Geometry check sheet. Reference: the model listing, model coordinates, mm. A direction names the side the tool comes from. Coordinates: 2 decimals unless noted, no trailing zeros. Write each loop counter-clockwise with the first axis right and the second up, starting at its lowest first coordinate (ties: lowest second). Pieces come first, ordered by that corner, then holes. Notation, with made-up numbers: (39.5, 14.25) -> (76.5, 14.25) arc R7 ccw to (76.5, 23.25) -> close; hole circle Ø4 at (80.25, -14). An arc over 180 degrees is marked (long way). Answer in a Markdown table with one row per item. Add a question column.
Q1. Gauge pin test, flat ends, axial feed: P1, Ø1.8, axis at x = 10, z = -3.5, coming from the -Y side; P2, Ø5, axis at x = 7.5, y = 9, coming from the -Z side; P3, Ø5, axis at x = 4, z = 3, coming from the -Y side. Record the tip position at first contact, or that the pin passes through.
Q2. Section check B-B, the plane z = -11. Record the boundary of the cut face in (x, y), and give its area (3 significant figures).
Q3. Tool access check on faces 1 (the face through (11, -4.65, -1)), 2 (the face through (6, -1.5, -25)), 3 (the face through (9.65, -6.79, -10.76)), 4 (the face through (6, 0, 2)), 5 (the face through (6, -1.5, 2)). Record the directions out of +Z, -Z, +X, -X, +Y, -Y that give a thin tool (end or side, any length) a straight path to the whole face; none if there is none.
Q4. Section check A-A, the plane x = 10.75. Record the boundary of the cut face in (y, z), and give its area (3 significant figures).
Q5. Section check C-C, the plane y = 13. Record the boundary of the cut face in (x, z), and give its area (3 significant figures).
Q6. Thickness scan on line 1 (Y direction, x = 7.75, z = -1.5); line 2 (Y direction, x = 9.5, z = -14); line 3 (Z direction, x = 3.75, y = -4.5). Record the ranges inside material, lowest first.
```python
from build123d import *

# Parameters (mm, degrees)
EXTRUDE_1_DEPTH = 12
SKETCH_2_R      = 6
EXTRUDE_2_DEPTH = 4.35
SKETCH_3_R      = 1.75
EXTRUDE_3_DEPTH = 4


with BuildPart() as part:
    # 草图1 → 凸台-拉伸1 (new body)
    with BuildSketch(Plane(origin=(0, 0, 0), x_dir=(0, 0, -1), z_dir=(1, 0, 0))):
        Polygon((0, 0), (0, 15), (23, 15), (23, 0), (27.4, 0), (27.4, -1.5), (23, -1.5), (23, -4.65), (0, -4.65), (0, -1.5), (-4.4, -1.5), (-4.4, 0), align=None)
    extrude(amount=EXTRUDE_1_DEPTH)

    # 草图2 → 凸台-拉伸2 (add)
    with BuildSketch(Plane(origin=(0, -4.65, 0), x_dir=(-1, 0, 0), z_dir=(0, -1, 0))):
        with Locations(Location((-6, 6, 0), (0, 0, 270))):
            Circle(SKETCH_2_R)
    extrude(amount=EXTRUDE_2_DEPTH)

    # 草图3 → 凸台-拉伸3 (add)
    with BuildSketch(Plane.XZ.offset(9)):
        with Locations(Location((6, -6, 0), (0, 0, 270))):
            Circle(SKETCH_3_R)
    extrude(amount=EXTRUDE_3_DEPTH)


solid = part.part
```
Calculated:
| question | item | result |
|---|---|---|
| 1 | P1 | stops at y = -9 |
| 1 | P2 | stops at z = -23 |
| 1 | P3 | stops at y = -1.5 |
| 2 | outline | (0, -4.65) -> (2.68, -4.65) -> (2.68, -9) -> (9.32, -9) -> (9.32, -4.65) -> (12, -4.65) -> (12, 15) -> (0, 15) -> close |
| 2 | area | 265 mm² |
| 3 | face 1 | +Z, +X, -Y |
| 3 | face 2 | -Z, +X, -X, -Y |
| 3 | face 3 | -Y |
| 3 | face 4 | +Z, +X, -X, +Y |
| 3 | face 5 | +Z, +X, -X, -Y |
| 4 | outline | (-9, -9.67) -> (-4.65, -9.67) -> (-4.65, -23) -> (-1.5, -23) -> (-1.5, -27.4) -> (0, -27.4) -> (0, -23) -> (15, -23) -> (15, 0) -> (0, 0) -> (0, 4.4) -> (-1.5, 4.4) -> (-1.5, 0) -> (-4.65, 0) -> (-4.65, -2.33) -> (-9, -2.33) -> close |
| 4 | area | 497 mm² |
| 5 | outline | (0, -23) -> (12, -23) -> (12, 0) -> (0, 0) -> close |
| 5 | area | 276 mm² |
| 6 | line 1 | y = -9 to 15 |
| 6 | line 2 | y = -4.65 to 15 |
| 6 | line 3 | z = -23 to 0 |
